Part print with two shaded views. Sizes in mm from the minimum x, y, z corner. Coordinates: 2 decimals unless noted, no trailing zeros. Order: outer loops, then holes, each group sorted by start corner. A loop starts at its lowest first (then second) coordinate and runs counter-clockwise, first axis right, second up. Notation, with made-up numbers: (2, 40) - (24, 40) arc R14 cw to (24, 52) - close; hole circle Ø1 at (-36.5, -36.5). An arc over 180 degrees is marked (long way). Write each question's results on one line, items separated by ' | '. Start each with the question number.
Q1. Band-saw the part on C-C, the plane y = 0.75. Write the cut outline in (x, z).
Q2. Band-saw the part on B-B, the plane x = 1.5. Write the cut outline in (y, z).
Q3. Wall check: probe 1 along X at (y, z) = (0.75, 0.15); probe 2 along Y at (x, z) = (1.65, 0.1); probe 3 along Y at (x, z) = (1.8, 0.15). Give the ranges that are in metal, low to high.
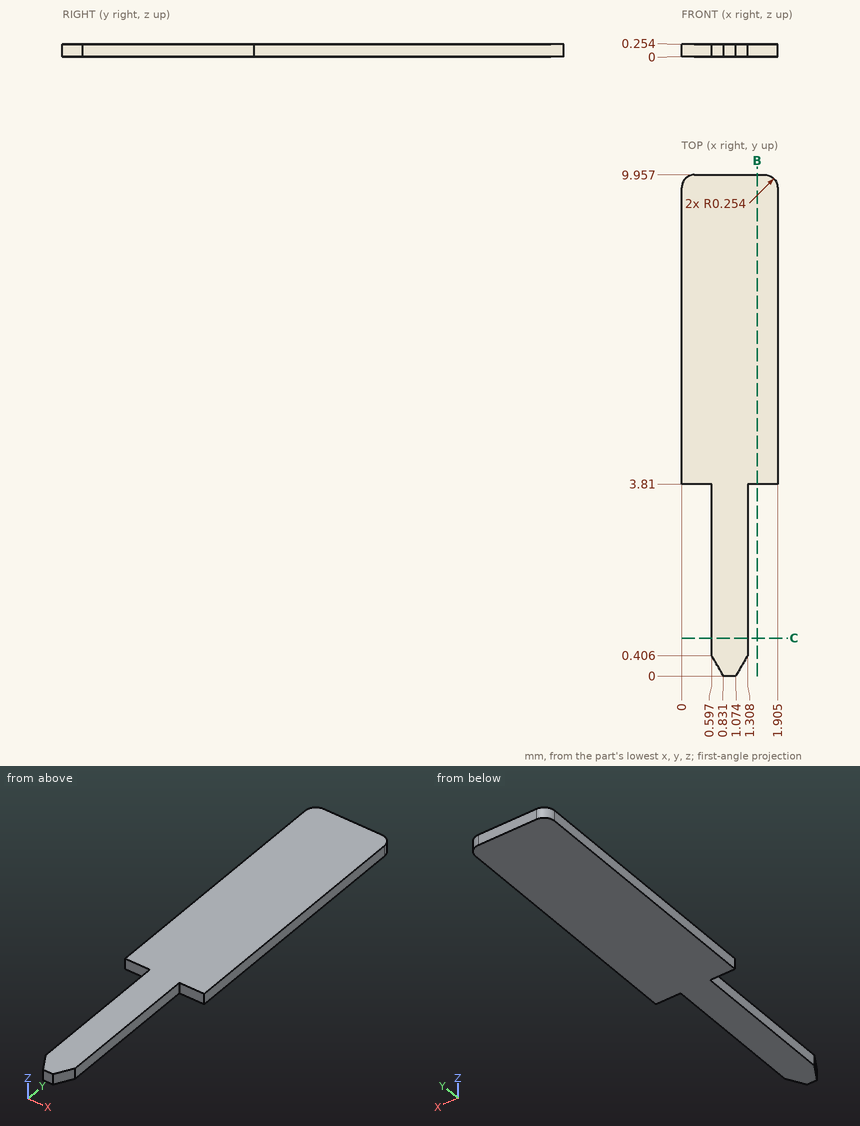
Results below:
1) outline: (0.6, 0) - (1.31, 0) - (1.31, 0.25) - (0.6, 0.25) - close
2) outline: (3.81, 0) - (9.96, 0) - (9.96, 0.25) - (3.81, 0.25) - close
3) probe 1: x = 0.6 to 1.31 | probe 2: y = 3.81 to 9.96 | probe 3: y = 3.81 to 9.91
